Job drawing, mm, ordinate dimensions from the low corner. One solid piece. A direction names the side the tool comes from. Round coordinates to 2 decimals unless told otherwise and drop trailing zeros. Loops run counter-clockwise (first coordinate to the right, second up) from the corner with the lowest first, then second, coordinate; pieces in that order, holes last. Notation, with made-up numbers: M 47.25,-13 L 101.25,-13 A15 cw 101.25,-1 Z; hole C 8,43.5 d8. An arc over 180 degrees is marked long. Use a Markdown table: item, result. Add a question column.
(1) Flat gauge pins, fed straight in: P1, Ø5, axis at x = 13.5, z = 15, coming from the +Y side; P2, Ø1.9, axis at x = 25, z = 11.9, coming from the -Y side (3 decimals); P3, Ø3, axis at y = 3, z = 4, coming from the +X side; P4, Ø7, axis at x = 24.5, z = 17.5, coming from the -Y side. Where does each tip first touch, or does it go through?
(2) Band-saw the part on C-C, the plane y = 5.6. Write the cut outline in (x, z), and give its area (3 significant figures).
(3) Band-saw the part on D-D, the plane x = 13.9. Write the cut outline in (y, z), and give its area (3 significant figures).
(4) Band-saw the part on B-B, the plane x = 2.8. Write the cut outline in (y, z), and give its area (3 significant figures).
(5) Two-plate mould, pull along X, no slides. Class the marked faces 1 and 2: released by +X, released by -X, zero draft, split by the parting line, or undercut.
(6) Which spindle directions (+Z, -Z, +X, -X, +Y, -Y) get a long thin tool onto all of the face, cutting with end or side? Do the marked faces 3, 4, 5, 6 and 7. Say none if no direction does.
(7) Band-saw the part on A-A, the plane z = 7. Write the cut outline in (x, y), and give its area (3 significant figures).
(8) Wall check: L1, parallel to X at y = 2.95, z = 17; L2, parallel to Y at x = 21.5, z = 21.75; L3, parallel to X at y = 1.2, z = 10.25. Give the ranges that are in metal, low to high.
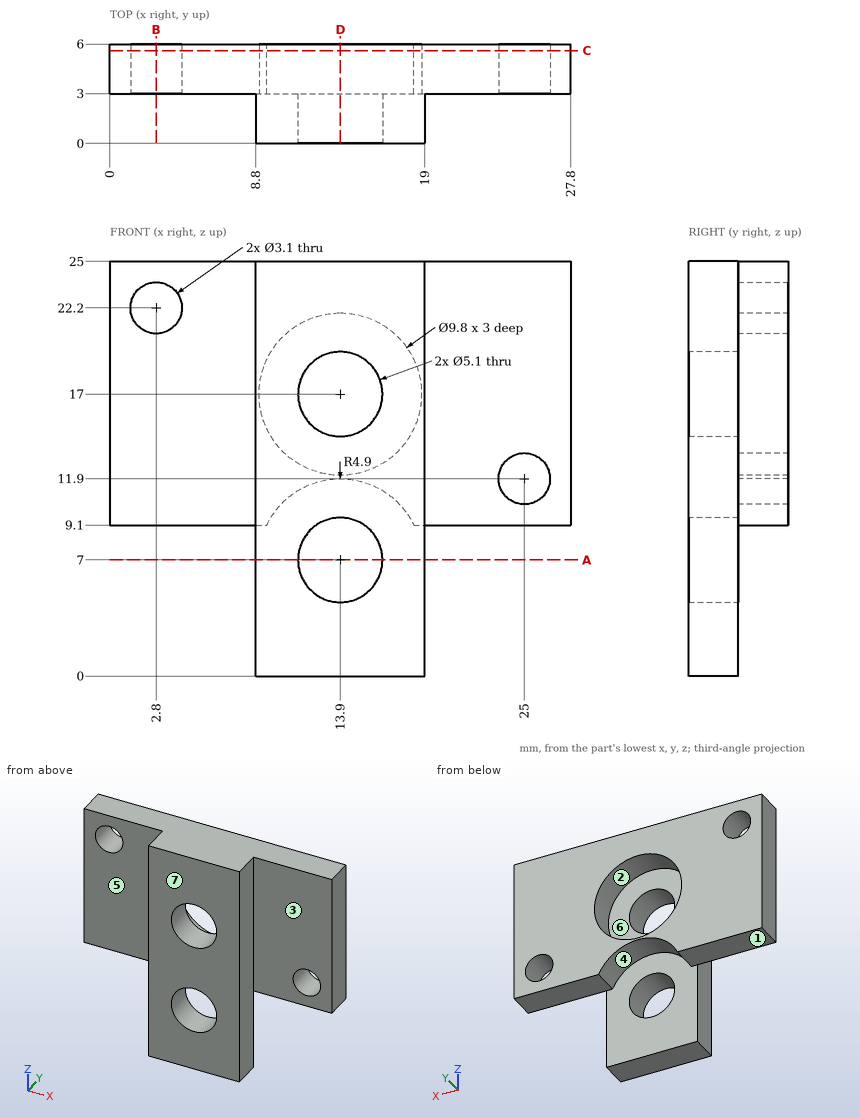
Return value:
| question | item | result |
|---|---|---|
| 1 | P1 | y = 3 |
| 1 | P2 | through |
| 1 | P3 | x = 19 |
| 1 | P4 | y = 3 |
| 2 | outline | M 0,9.1 L 9.47,9.1 A4.9 cw 18.33,9.1 L 27.8,9.1 L 27.8,25 L 0,25 Z; hole C 2.8,22.2 d3.1; hole C 13.9,17 d9.8; hole C 25,11.9 d3.1 |
| 2 | area | 334 mm^2 |
| 3 | outline | M 0,0 L 3,0 L 3,4.45 L 0,4.45 Z; M 0,9.55 L 3,9.55 L 3,11.9 L 6,11.9 L 6,12.1 L 3,12.1 L 3,14.45 L 0,14.45 Z; M 0,19.55 L 3,19.55 L 3,21.9 L 6,21.9 L 6,25 L 0,25 Z |
| 3 | area | 54.3 mm^2 |
| 4 | outline | M 3,9.1 L 6,9.1 L 6,20.65 L 3,20.65 Z; M 3,23.75 L 6,23.75 L 6,25 L 3,25 Z |
| 4 | area | 38.4 mm^2 |
| 5 | face 1 | zero draft |
| 5 | face 2 | undercut |
| 6 | face 3 | +Z, -Z, +X, -Y |
| 6 | face 4 | -Z, +Y |
| 6 | face 5 | +Z, -Z, -X, -Y |
| 6 | face 6 | +Y |
| 6 | face 7 | +Z, -Z, +X, -X, -Y |
| 7 | outline | M 8.8,0 L 11.35,0 L 11.35,3 L 8.8,3 Z; M 16.45,0 L 19,0 L 19,3 L 16.45,3 Z |
| 7 | area | 15.3 mm^2 |
| 8 | L1 | 8.8 to 11.35, 16.45 to 19 |
| 8 | L2 | 3 to 6 |
| 8 | L3 | 8.8 to 19 |
